Study the drawing (mm; zero at the part's minimum x, y, z) and answer. A direction names the side the tool comes from. Coordinates: 2 decimals unless noted, no trailing zeros. Write each loop counter-clockwise with the first axis right and the second up, starting at its lowest first coordinate (ties: lowest second). Pieces come first, ordered by that corner, then holes. Notation, with made-up numbers: M 1,29.25 L 34,29.25 A22 cw 34,54.25 Z; hole C 75,58.5 d3. An arc over 180 degrees is marked long. Answer as CSV lines item,"result". Start each with the question number.
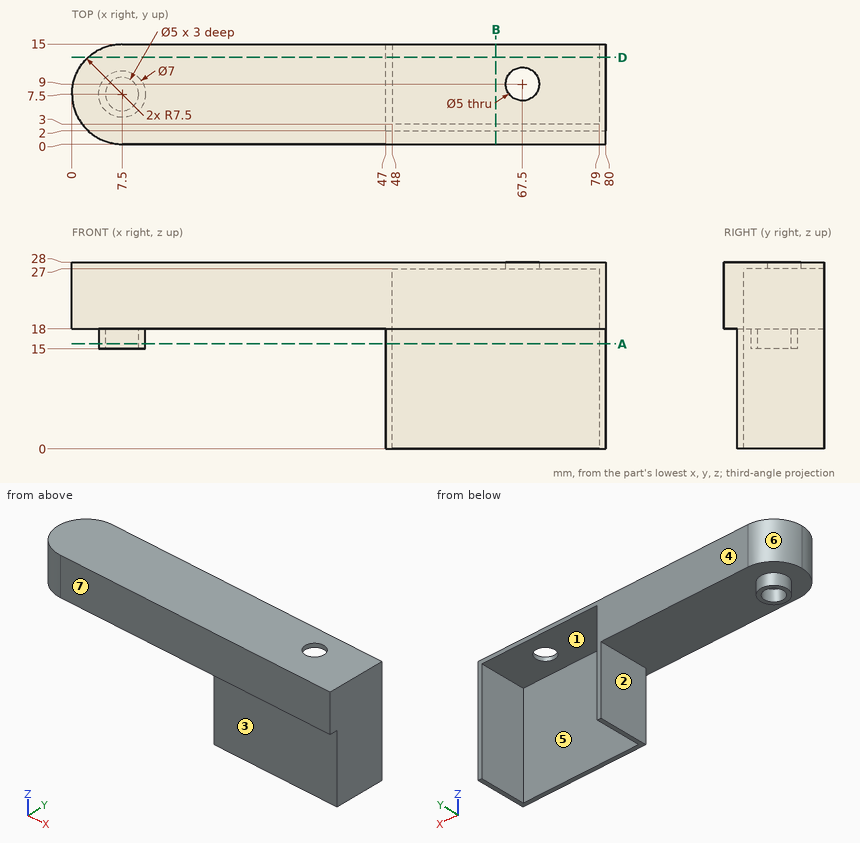
1) The part is cut by section A-A (z = 15.75). Determine the outline of the cut face in (x, y).
2) Which of the six approach directions +Z, -Z, +X, -X, +Y, -Y give full straight-line access (tool end or side, diameter ignored) to the marked faces 1, 2, 3 and 4?
3) The part is cut by section B-B (x = 63.5). Determine the outline of the cut face in (y, z).
4) Find the intervals of material crossed by line 1 (Y direction, x = 7.5, z = 16.65); line 2 (Y direction, x = 67.5, z = 27.3); line 3 (Z direction, x = 4.5, y = 4.75), in increasing order. Write a range as from..to.
5) For a pull along X with two mould halves and no side action, classify the marked faces 5, 6 and 7 as +X half, -X half, draft (parallel to the pull), parting line (faces both ways), or undercut.
6) The part is cut by section D-D (y = 13). Determine the outline of the cut face in (x, z), then the cut area to 3 significant figures.
7) Each of these flat-tipped pins is pushed along its axis until it touches: P1, Ø8, axis at x = 64.5, z = 18.5, coming from the +Y side; P2, Ø1, axis at x = 47, z = 9, coming from the -Y side; P3, Ø2, axis at y = 12.5, z = 14, coming from the -X side. Where does it stop, or does it pass through?
Completed:
1,outline,"C 7.5,7.5 d7; M 47,2 L 80,2 L 80,15 L 79,15 L 79,3 L 48,3 L 48,15 L 47,15 Z; hole C 7.5,7.5 d5"
2,face 1,"-Z, +Y"
2,face 2,"-Z, +Y, -Y"
2,face 3,"-Z, +X, -X, -Y"
2,face 4,"+Z, -Z, +X, -X, +Y"
3,outline,"M 0,18 L 2,18 L 2,0 L 3,0 L 3,27 L 15,27 L 15,28 L 0,28 Z"
4,line 1,"4..5, 10..11"
4,line 2,"0..6.5, 11.5..15"
4,line 3,"18..28"
5,face 5,"undercut"
5,face 6,"-X half"
5,face 7,"draft"
6,outline,"M 2.4,18 L 47,18 L 47,0 L 48,0 L 48,27 L 79,27 L 79,0 L 80,0 L 80,28 L 2.4,28 Z"
6,area,"533 mm²"
7,P1,"y = 3"
7,P2,"y = 2"
7,P3,"x = 47"
